The model under review builds one solid part; all positions refer to its coordinate system, in mm. Face numbers are marked on the shaded views. A direction names the side the tool comes from. Round coordinates to 2 decimals unless told otherwise and drop trailing zeros. Order: outer loops, then holes, each group sorted by start corner. A loop starts at its lowest first (then second) coordinate and runs counter-clockwise, first axis right, second up. Notation, with made-up numbers: (77.5, 48) -> (97.5, 48) arc R30 ccw to (97.5, 72) -> close; hole circle Ø2 at (11, -22). An arc over 180 degrees is marked (long way). Put each result on its own line as item: value. Start each with the question number.
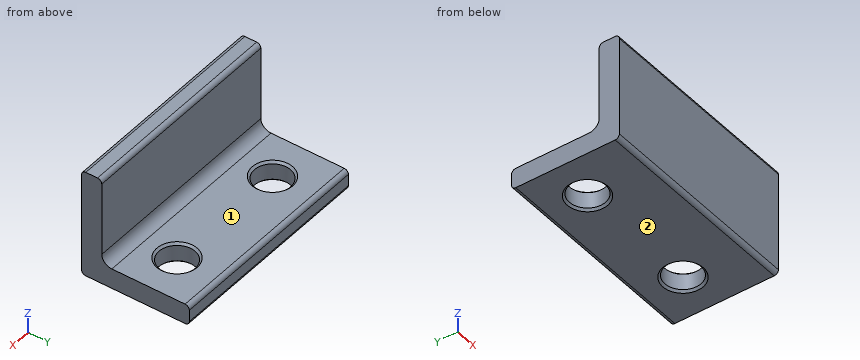
from build123d import *

# Parameters (mm, degrees)
F1_DEPTH = 25
F2_R     = 1
F3_R     = 2.38125
F4_R     = 4.25
F5_DEPTH = 25
F6_SIZE  = 0.5
F7_R     = 2.5
F8_DEPTH = 25


with BuildPart() as f1:
    # F0 (on Right) → F1 (new body, symmetric)
    with BuildSketch(Plane.YZ):
        Polygon((0, 25.4), (0, 0), (25.4, 0), (25.4, 4.7625), (4.7625, 4.7625), (4.7625, 25.4), align=None)
    extrude(amount=F1_DEPTH, both=True)

    # F2
    f2_edges = [f1.edges().sort_by_distance(p)[0] for p in [
        (0, 0, 25.4),
        (0, 4.7625, 25.4),
        (0, 0, 0),
        (0, 25.4, 4.7625),
        (0, 25.4, 0),
    ]]
    fillet(f2_edges, radius=F2_R)

    # F3
    f3_edges = [f1.edges().sort_by_distance(p)[0] for p in [
        (0, 4.7625, 4.7625),
    ]]
    fillet(f3_edges, radius=F3_R)

    # F4 (on face) → F5 (cut)
    with BuildSketch(Plane.XY.offset(4.7625)):
        with Locations((-15, 15)):
            Circle(F4_R)
        with Locations((715, 15)):
            Circle(F4_R)
        with Locations((1445, 15)):
            Circle(F4_R)
        with Locations((15, 15)):
            Circle(F4_R)
    extrude(amount=-F5_DEPTH, mode=Mode.SUBTRACT)

    # F6
    f6_edges = [f1.edges().sort_by_distance(p)[0] for p in [
        (-19.25, 15, 4.7625),
        (-10.75, 15, 2.38125),
        (-19.25, 15, 0),
        (10.75, 15, 4.7625),
        (19.25, 15, 2.38125),
        (10.75, 15, 0),
    ]]
    chamfer(f6_edges, length=F6_SIZE)

    # F7 (on face) → F8 (cut)
    with BuildSketch(Plane.XZ):
        with Locations((65, 20)):
            Circle(F7_R)
        with Locations((-65, 20)):
            Circle(F7_R)
    extrude(amount=-F8_DEPTH, mode=Mode.SUBTRACT)


solid = f1.part
Q1. Take a section at C-C on x = -4. Give the boundary of the cut face in (y, z).
Q2. Take a section at A-A on y = 15. Give the boundary of the cut face in (x, z).
Q3. Take a section at D-D on y = 23.5. Give the boundary of the cut face in (x, z), and give its area (3 significant figures).
Q4. For the marked faces 1 and 2, list the 3-axis set-ups (+Z, -Z, +X, -X, +Y, -Y) from which the entire face can be reached by the end or side of a thin tool; tool diameter is ignored.
Q5. Take a section at B-B on x = 15. Give the boundary of the cut face in (y, z).
Q6. Wall thickness on probe 1 along Y at (x, z) = (-15, 2.3); probe 2 along Z at (x, y) = (18, 10.25): over which ranges is each line inside the solid? List them lowest first. Write a range as [from, to].
Q7. Clearance check with flat-ended pins moving along their axes: pin 1 Ø4 at (y, z) = (14.5, 5) entering from +X; pin 2 Ø14 at (x, z) = (7, 16.5) entering from +Y. State where each tip first meets the part, or that it passes through.
Calculated:
1. outline: (0, 1) arc R1 ccw to (1, 0) -> (24.4, 0) arc R1 ccw to (25.4, 1) -> (25.4, 3.76) arc R1 ccw to (24.4, 4.76) -> (7.14, 4.76) arc R2.38 cw to (4.76, 7.14) -> (4.76, 24.4) arc R1 ccw to (3.76, 25.4) -> (1, 25.4) arc R1 ccw to (0, 24.4) -> close
2. outline: (-25, 0) -> (-19.75, 0) -> (-19.25, 0.5) -> (-19.25, 4.26) -> (-19.75, 4.76) -> (-25, 4.76) -> close; (-10.75, 0.5) -> (-10.25, 0) -> (10.25, 0) -> (10.75, 0.5) -> (10.75, 4.26) -> (10.25, 4.76) -> (-10.25, 4.76) -> (-10.75, 4.26) -> close; (19.25, 0.5) -> (19.75, 0) -> (25, 0) -> (25, 4.76) -> (19.75, 4.76) -> (19.25, 4.26) -> close
3. outline: (-25, 0) -> (25, 0) -> (25, 4.76) -> (-25, 4.76) -> close
3. area: 238 mm²
4. face 1: +Z, +X, -X, +Y
4. face 2: -Z, +X, -X, +Y, -Y
5. outline: (0, 1) arc R1 ccw to (1, 0) -> (10.25, 0) -> (10.75, 0.5) -> (10.75, 4.26) -> (10.25, 4.76) -> (7.14, 4.76) arc R2.38 cw to (4.76, 7.14) -> (4.76, 24.4) arc R1 ccw to (3.76, 25.4) -> (1, 25.4) arc R1 ccw to (0, 24.4) -> close; (19.25, 0.5) -> (19.75, 0) -> (24.4, 0) arc R1 ccw to (25.4, 1) -> (25.4, 3.76) arc R1 ccw to (24.4, 4.76) -> (19.75, 4.76) -> (19.25, 4.26) -> close
6. probe 1: y = [0, 10.75], [19.25, 25.4]
6. probe 2: z = [0, 4.76]
7. pin 1: stops at x = 25
7. pin 2: stops at y = 4.76
